The listing builds one solid part. Answer for the finished solid, in the listing's coordinates (mm). Face numbers are marked on the shaded views. A direction names the side the tool comes from. Coordinates: 2 decimals unless noted, no trailing zeros. Order: outer loops, then holes, each group sorted by start corner. A loop starts at its lowest first (then second) coordinate and runs counter-clockwise, first axis right, second up.
```python
from build123d import *

# Parameters (mm, degrees)
F0_W     = 96.55572474
F0_H     = 63.9681667089
F1_DEPTH = 76.2
F2_R     = 4.9691003704
F3_DEPTH = 50.8
F4_SIZE  = 5.08
F5_SIZE  = 5.08
F6_D     = 12.7
F7_D     = 6.35
F8_R     = 5.08
F9_R     = 5.08
F10_D    = 25.4


with BuildPart() as f1:
    # F0 (on Front) → F1 (new body)
    with BuildSketch(Plane.XZ):
        with Locations((0, 31.6823422909)):
            Rectangle(F0_W, F0_H)
    extrude(amount=F1_DEPTH)

    # F2 (on face) → F3 (join)
    with BuildSketch(Plane.XZ.offset(76.2)):
        with Locations((0, 31.6823422909)):
            Circle(F2_R)
    extrude(amount=F3_DEPTH)

    # F4
    f4_edges = [f1.edges().sort_by_distance(p)[0] for p in [
        (48.277862, -76.2, 31.682342),
        (0, -76.2, -0.301741),
        (0, -76.2, 63.666426),
        (-48.277862, -76.2, 31.682342),
        (-4.9691, -76.2, 31.682342),
    ]]
    chamfer(f4_edges, length=F4_SIZE)

    # F5
    f5_edges = [f1.edges().sort_by_distance(p)[0] for p in [
        (48.277862, 0, 31.682342),
        (0, 0, 63.666426),
        (-48.277862, 0, 31.682342),
        (0, 0, -0.301741),
    ]]
    chamfer(f5_edges, length=F5_SIZE)

    # F6 (through all)
    with Locations(Plane(origin=(0, 0, 0), x_dir=(1, 0, 0), z_dir=(0, 1, 0))):
        with Locations((-29.6028293669, -33.6742401123)):
            Hole(F6_D / 2)

    # F7 (through all)
    with Locations(Plane(origin=(0, 0, 0), x_dir=(1, 0, 0), z_dir=(0, 1, 0))):
        with Locations((0, -31.6823422909)):
            Hole(F7_D / 2)

    # F8
    f8_edges = [f1.edges().sort_by_distance(p)[0] for p in [
        (-48.277862, -38.1, -0.301741),
    ]]
    fillet(f8_edges, radius=F8_R)

    # F9
    f9_edges = [f1.edges().sort_by_distance(p)[0] for p in [
        (48.277862, -38.1, -0.301741),
        (48.277862, -38.1, 63.666426),
        (-48.277862, -38.1, 63.666426),
    ]]
    fillet(f9_edges, radius=F9_R)

    # F10 (through all)
    with Locations(Plane(origin=(0, 0, 0), x_dir=(1, 0, 0), z_dir=(0, 1, 0))):
        with Locations((28.7802238017, -36.0331609845)):
            Hole(F10_D / 2)


solid = f1.part
```
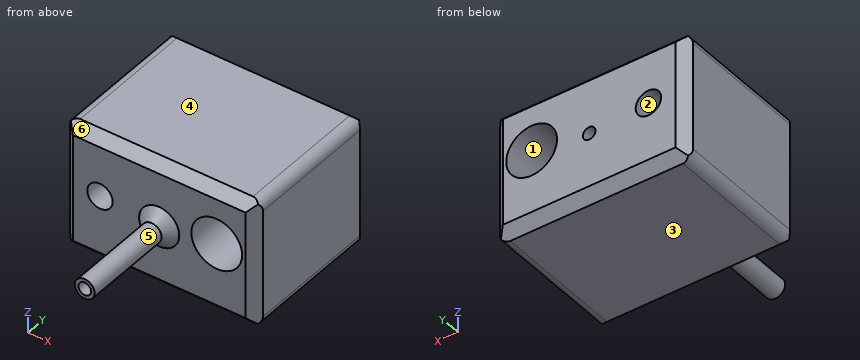
(1) Find section A-A (x = 0). Write down the section's boundary in (y, z), and give its area (3 significant figures).
(2) This flat-tipped pin is pushed along its axis until it touches: pin 1 Ø12 at (x, z) = (-8, 7.5) entering from -Y. Where does it stop, or does it pass through?
(3) Find section C-C (y = -50). Write down the section's boundary in (x, z) (3 decimals).
(4) Find section D-D (z = 45). Write down the section's boundary in (x, y).
(5) Find section B-B (z = 18). Write down the section's boundary in (x, y).
(6) Consider line 1 (Z direction, x = 0, y = -36); line 2 (X direction, y = -57, z = 35); line 3 (Y direction, x = 40.5, z = 20). Determine where each line is inside the solid, lowest interval first.
(7) For the marked faces 5 and 6, determine the directions among +Z, -Z, +X, -X, +Y, -Y from which every point of the face is accessible in a straight line to the end or side of a thin tool.
(8) The mould has two halves that part along Z. Classify the marked faces 1, 2, 3 and 4: released by +Z, released by -Z, zero draft, split by the parting line, or undercut.
Findings below:
1. outline: (-127, 26.71) - (-81.28, 26.71) - (-76.2, 21.63) - (-76.2, 4.78) - (-71.12, -0.3) - (-5.08, -0.3) - (0, 4.78) - (0, 28.51) - (-127, 28.51) - close; (-127, 34.86) - (0, 34.86) - (0, 58.59) - (-5.08, 63.67) - (-71.12, 63.67) - (-76.2, 58.59) - (-76.2, 41.73) - (-81.28, 36.65) - (-127, 36.65) - close
1. area: 4,550 mm2
2. pin 1: stops at y = -76.2
3. outline: (-48.278, 4.778) arc R5.08 ccw to (-43.198, -0.302) - (43.198, -0.302) arc R5.08 ccw to (48.278, 4.778) - (48.278, 58.586) arc R5.08 ccw to (43.198, 63.666) - (-43.198, 63.666) arc R5.08 ccw to (-48.278, 58.586) - close; hole circle Ø12.7 at (-29.603, 33.674); hole circle Ø6.35 at (0, 31.682); hole circle Ø25.4 at (28.78, 36.033)
4. outline: (-48.28, -71.12) - (-43.2, -76.2) - (19.79, -76.2) - (19.79, 0) - (-43.2, 0) - (-48.28, -5.08) - close; (37.77, -76.2) - (43.2, -76.2) - (48.28, -71.12) - (48.28, -5.08) - (43.2, 0) - (37.77, 0) - close
5. outline: (-48.28, -71.12) - (-43.2, -76.2) - (43.2, -76.2) - (48.28, -71.12) - (48.28, -5.08) - (43.2, 0) - (-43.2, 0) - (-48.28, -5.08) - close
6. line 1: z = -0.3 to 28.51, 34.86 to 63.67
6. line 2: x = -48.28 to -35.81, -23.39 to 16.12, 41.44 to 48.28
6. line 3: y = -76.2 to 0
7. face 5: -Y
7. face 6: +Z, +X, -X, -Y
8. face 1: undercut
8. face 2: undercut
8. face 3: released by -Z
8. face 4: released by +Z
